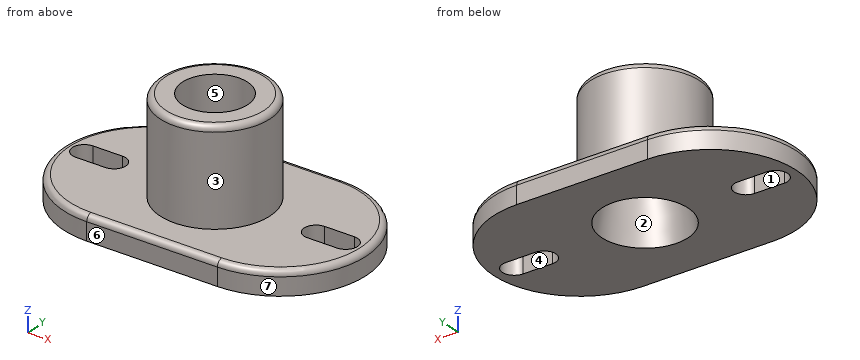
Autodesk Inventor part; units mm, degrees
ref_plane "작업 평면1" through (-22, 0, 0) normal (0, 1, 0) x (1, 0, 0)
ref_plane "YZ Plane" through (0, 0, 0) normal (1, 0, 0) x (0, 1, 0)
ref_plane "XZ Plane" through (0, 0, 0) normal (0, 1, 0) x (-1, 0, 0)
sketch "스케치1" plane through (0, 0, 0) normal (0, 0, 1) x (1, 0, 0)
  line L0 (-22, 0) -> (22, 0) construction
  line L1 (-22, -29) -> (22, -29)
  line L2 (22, 29) -> (-22, 29)
  arc A0 (-22, 29) -> (-22, -29) centre (-22, 0) ccw
  arc A1 (22, -29) -> (22, 29) centre (22, 0) ccw
  line L3 (-44, 0) -> (-34, 0) construction
  line L4 (-44, -4) -> (-34, -4)
  line L5 (-34, 4) -> (-44, 4)
  arc A2 (-44, 4) -> (-44, -4) centre (-44, 0) ccw
  arc A3 (-34, -4) -> (-34, 4) centre (-34, 0) ccw
  line L6 (44, 0) -> (34, 0) construction
  line L7 (44, 4) -> (34, 4)
  line L8 (34, -4) -> (44, -4)
  arc A4 (44, -4) -> (44, 4) centre (44, 0) ccw
  arc A5 (34, 4) -> (34, -4) centre (34, 0) ccw
  circle A6 centre (0, 0) radius 18.5
  circle A7 centre (0, 0) radius 11
  point P0 (-39, 0)
  point P1 (39, 0)
  dimension "d0" = 29
  dimension "d1" = 102
  dimension "d2" = 10
  dimension "d3" = 8
  dimension "d4" = 10
  dimension "d5" = 8
  dimension "d6" = 68
  dimension "d7" = 34
  dimension "d8" = 37
  dimension "d9" = 22
extrude "돌출1" add sketch "스케치1" along normal blind 8 contours A0 L2 A1 L1
extrude "돌출2" add sketch "스케치1" along normal blind 40 contours A6
ref_plane "작업 평면1" through (-22, 0, 0) normal (0, 1, 0) x (1, 0, 0)
sketch "스케치2" plane through (-22, 0, 0) normal (0, 1, 0) x (1, 0, 0)
  line L0 (36.5, 0) -> (34.1671, -19)
  line L1 (34.1671, -19) -> (9.8329, -19)
  line L2 (33, -40) -> (33, 0)
  line L3 (9.8329, -19) -> (7.5, 0)
  line L4 (85.0441, 0) -> (-77.2032, 0)
  line L5 (22, 10.7301) -> (22, -88.2666)
  point P0 (22, 0)
  point P1 (22, 0)
  point P2 (22, 0)
  point P3 (22, -19)
  dimension "d14" = 14
  dimension "d16" = 29
  dimension "d17" = 19
  dimension "d18" = 19
  dimension "d19" = 0
  dimension "d20" = 0
  dimension "d21" = 14.5
revolve "회전1" cut sketch "스케치2" angle 360 about axis through (0, 0, -10.7301) along (0, 0, 1) contours L0 L1 L2 L4 | L2 L1 L5 L4
fillet "모깎기1" radius 2 1 edges at (-12.1671, 0, 19)
fillet "모깎기2" radius 2 5 edges at (-18.5, 0, 40) (0, -29, 8) (51, 0, 8) (0, 29, 8) (-51, 0, 8)
properties part number "부품1"
Read the model definition and answer for the solid it produces. Units are mm, in the model's axes. Face numbers are marked on the shaded views. A direction names the side the tool comes from. Coordinates: 2 decimals unless noted, no trailing zeros. Order: outer loops, then holes, each group sorted by start corner. A loop starts at its lowest first (then second) coordinate and runs counter-clockwise, first axis right, second up. Notation, with made-up numbers: (85, 76.5) - (133, 76.5) arc R20 ccw to (133, 83.5) - close; hole circle Ø10 at (-11.5, 59.25). An arc over 180 degrees is marked (long way). Answer as a JSON object with one key per item and string values. Group by question number.
Item 1: A tool of negligible diameter and unlimited length cuts with its end or side. For the marked faces 1, 2 and 3, from which of +Z, -Z, +X, -X, +Y, -Y can it reach the whole face along a straight path? Write none if from no direction.
Item 2: Flat-ended cylindrical pins translate along their axes: P1, Ø10, axis at x = -13, z = 12, coming from the -Y side; P2, Ø4, axis at x = 17.5, y = -9, coming from the +Z side; P3, Ø6.5, axis at x = -38.5, z = 2, coming from the +Y side. Find the tip coordinate at first contact, or state that the pin passes through.
Item 3: Section B-B (y = 0) is taken. Give the vertices of the cut face in (x, z).
Item 4: Consider probe 1 along Y at (x, z) = (0, 34.5); probe 2 along Z at (x, y) = (30.5, -5); probe 3 along Z at (x, y) = (-10, 13.5). Determine where each line is inside the solid, lowest interval first. Write a range as from..to.
Item 5: Section D-D (x = 21) is taken. Give the vertices of the cut face in (y, z).
Item 6: The mould has two halves that part along Y. Classify the marked faces 4, 5, 6 and 7: +Y half, -Y half, draft (parallel to the pull), parting line (faces both ways), or undercut.
Item 7: Section A-A (x = 0) is taken. Give the vertices of the cut face in (y, z), plus the area to 3 significant figures.
Item 8: Section C-C (z = 3) is taken. Give the vertices of the cut face in (x, y), plus the area to 3 significant figures.
Results are:
{
 "1": {"face 1": "+Z, -Z", "face 2": "-Z", "face 3": "+Z"},
 "2": {"P1": "stops at y = -28.73", "P2": "stops at z = 39.62", "P3": "stops at y = 25.8"},
 "3": {"outline": "(-51, 0) - (-48, 0) - (-48, 8) - (-49, 8) arc R2 ccw to (-51, 6) - close; (-30, 0) - (-14.5, 0) - (-12.37, 17.34) arc R2 cw to (-11, 19) - (-11, 40) - (-16.5, 40) arc R2 ccw to (-18.5, 38) - (-18.5, 8) - (-30, 8) - close; (11, 19) arc R2 cw to (12.37, 17.34) - (14.5, 0) - (30, 0) - (30, 8) - (18.5, 8) - (18.5, 38) arc R2 ccw to (16.5, 40) - (11, 40) - close; (48, 0) - (51, 0) - (51, 6) arc R2 ccw to (49, 8) - (48, 8) - close"},
 "4": {"probe 1": "y = -18.5..-11, 11..18.5", "probe 2": "z = 0..8", "probe 3": "z = 0..39.98"},
 "5": {"outline": "(-29, 0) - (29, 0) - (29, 6) arc R2 ccw to (27, 8) - (-27, 8) arc R2 ccw to (-29, 6) - close"},
 "6": {"face 4": "undercut", "face 5": "undercut", "face 6": "-Y half", "face 7": "parting line"},
 "7": {"outline": "(-29, 0) - (-14.5, 0) - (-12.37, 17.34) arc R2 cw to (-11, 19) - (-11, 40) - (-16.5, 40) arc R2 ccw to (-18.5, 38) - (-18.5, 8) - (-27, 8) arc R2 ccw to (-29, 6) - close; (11, 19) arc R2 cw to (12.37, 17.34) - (14.5, 0) - (29, 0) - (29, 6) arc R2 ccw to (27, 8) - (18.5, 8) - (18.5, 38) arc R2 ccw to (16.5, 40) - (11, 40) - close", "area": "677 mm^2"},
 "8": {"outline": "(-22, -29) - (22, -29) arc R29 ccw to (22, 29) - (-22, 29) arc R29 ccw to start; hole (-44, -4) - (-34, -4) arc R4 ccw to (-34, 4) - (-44, 4) arc R4 ccw to start; hole circle Ø28.26 at (0, 0); hole (34, -4) - (44, -4) arc R4 ccw to (44, 4) - (34, 4) arc R4 ccw to start", "area": "4,310 mm^2"}
}
